Autodesk Inventor part; units mm, degrees
ref_plane "YZ Plane" through (0, 0, 0) normal (1, 0, 0) x (0, 1, 0)
ref_plane "XZ Plane" through (0, 0, 0) normal (0, 1, 0) x (-1, 0, 0)
ref_plane "XY Plane" through (0, 0, 0) normal (0, 0, 1) x (1, 0, 0)
sketch "Náčrt1" plane through (0, 0, 0) normal (0, 0, 1) x (1, 0, 0)
  line L0 (-25, 25) -> (25, 25)
  line L1 (25, 25) -> (25, -25)
  line L2 (25, -25) -> (-25, -25)
  line L3 (-25, -25) -> (-25, 25)
  line L4 (-25, 25) -> (25, -25) construction
  line L5 (25, 25) -> (-25, -25) construction
  line L6 (-25, 8.7) -> (-8.7, 25)
  circle A0 centre (-20, -20) radius 2.1
  circle A1 centre (20, 20) radius 2.1
  point P0 (0, 0)
  dimension "d0" = 50
  dimension "d1" = 50
  dimension "d2" = 33.7
  dimension "d3" = 45
  dimension "d4" = 4.2
  dimension "d6" = 5
  dimension "d7" = 5
extrude "Vysunutí1" add sketch "Náčrt1" along normal mid plane 18 contours L0 L1 L2 L3 L6
properties part number "Sensor"
The model under review builds one solid part; all positions refer to its coordinate system, in mm. Round coordinates to 2 decimals unless told otherwise and drop trailing zeros. Loops run counter-clockwise (first coordinate to the right, second up) from the corner with the lowest first, then second, coordinate; pieces in that order, holes last. Notation, with made-up numbers: M 49,15.5 L 76,15.5 A36 ccw 76,54.5 Z; hole C 44,32 d6. An arc over 180 degrees is marked long. Answer as a JSON object with one key per item and string values.
(1) Draft analysis for pull direction X (two halves, no side actions). For faces 1 (the flat face through (-25, -8, 0)), 2 (the cylindrical face through (-17.997, -20.631, -0.126)), 3 (the flat face through (0, 0, -9)), state which applies: released by +X, released by -X, zero draft, split by the parting line, or undercut.
Resolved:
{"face 1": "released by -X", "face 2": "undercut", "face 3": "zero draft"}
(2) Take a section at C-C on z = 7.25. Give the boundary of the cut face in (x, y).
Resolved:
{"outline": "M -25,-25 L 25,-25 L 25,25 L -8.7,25 L -25,8.7 Z; hole C -20,-20 d4.2; hole C 20,20 d4.2"}
(3) Take a section at B-B on y = -20. Give the boundary of the cut face in (x, z), and give its area (3 significant figures).
Resolved:
{"outline": "M -25,-9 L -22.1,-9 L -22.1,9 L -25,9 Z; M -17.9,-9 L 25,-9 L 25,9 L -17.9,9 Z", "area": "824 mm²"}
(4) Take a section at D-D on y = 14. Give the boundary of the cut face in (x, z), and give its area (3 significant figures).
Resolved:
{"outline": "M -19.7,-9 L 25,-9 L 25,9 L -19.7,9 Z", "area": "805 mm²"}
(5) Take a section at A-A on x = -20. Give the boundary of the cut face in (y, z), and give its area (3 significant figures).
Resolved:
{"outline": "M -25,-9 L -22.1,-9 L -22.1,9 L -25,9 Z; M -17.9,-9 L 13.7,-9 L 13.7,9 L -17.9,9 Z", "area": "621 mm²"}
(6) Clearance check with a flat-ended pin moving along its axis: P1, Ø2, axis at x = -14, z = 3, coming from the +Y side. State where the tip first meets the part, or that it passes through.
Resolved:
{"P1": "y = 20.7"}
(7) To check wall thickness, follow line 1 along Y through (x, z) = (20, -2.25); line 2 along Y through (x, z) = (21.5, -6); line 3 along Y through (x, z) = (-10.5, 7.75). State the ranges of each line that lie inside material, in increasing order.
Resolved:
{"line 1": "-25 to 17.9, 22.1 to 25", "line 2": "-25 to 18.53, 21.47 to 25", "line 3": "-25 to 23.2"}
